```python
from build123d import *

# Parameters (mm, degrees)
F0_R          = 2.5144921482
F0_R_2        = 19.25
F1_DEPTH      = 5
F4_END_RADIUS = 19.25
F4_REACH      = 78.1652482066


with BuildPart() as f1:
    # F0 (on Front) → F1 (new body)
    with BuildSketch(Plane.XZ):
        with BuildLine():
            Line((-27.2, -28.2), (27.2, -28.2))
            ThreePointArc((27.2, -28.2), (27.9071067812, -27.9071067812), (28.2, -27.2))
            Line((28.2, -27.2), (28.2, 27.2))
            ThreePointArc((28.2, 27.2), (27.9071067812, 27.9071067812), (27.2, 28.2))
            Line((27.2, 28.2), (-27.2, 28.2))
            ThreePointArc((-27.2, 28.2), (-27.9071067812, 27.9071067812), (-28.2, 27.2))
            Line((-28.2, 27.2), (-28.2, -27.2))
            ThreePointArc((-28.2, -27.2), (-27.9071067812, -27.9071067812), (-27.2, -28.2))
        make_face()
        with Locations((-23.57, -23.57)):
            Circle(F0_R, mode=Mode.SUBTRACT)
        with Locations((23.57, -23.57)):
            Circle(F0_R, mode=Mode.SUBTRACT)
        with Locations((-23.57, 23.57)):
            Circle(F0_R, mode=Mode.SUBTRACT)
        Circle(F0_R_2, mode=Mode.SUBTRACT)
        with Locations((23.57, 23.57)):
            Circle(F0_R, mode=Mode.SUBTRACT)
    extrude(amount=F1_DEPTH)

    f4_end = (Plane.ZX.offset(-2.5) * Cylinder(F4_END_RADIUS, 316.1669127895, mode=Mode.PRIVATE)).faces().sort_by_distance((-19.25, -2.5, 0))[0]
    # F3 (on face) → F4 (join, up to the whole of a round face its end follows)
    with BuildSketch(Plane(origin=(-28.2, 0, 0), x_dir=(0, -1, 0), z_dir=(-1, 0, 0))):
        Polygon((4.9999998882, -16.2), (4.9999998882, -19.2), (22.1499998882, -19.2), (22.1499998882, -16.2), (21.9999998882, -16.2), (16.7999998882, -16.2), (16.7999998882, -8.8), (22.1499998882, -8.8), (22.1499998882, -5.8), (4.9999998882, -5.8), align=None)
    f4_long = extrude(amount=-F4_REACH, mode=Mode.PRIVATE)
    add(split(f4_long, bisect_by=f4_end, keep=Keep.ALL, mode=Mode.PRIVATE).solids().sort_by_distance((-28.2, -12.347048043, -12.5))[0])

    # F5: F1 across plane


with BuildPart() as f1_1:
    add(f1.part)
    add(f1.part.mirror(Plane.YZ))


solid = f1_1.part
```
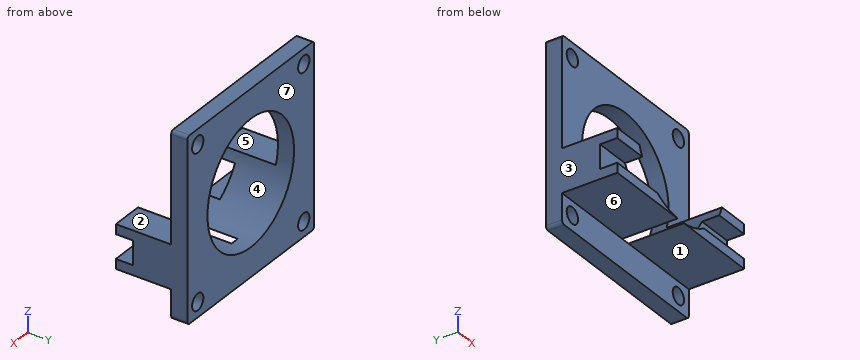
Model file for the job. Use its own axes, mm. Face numbers are marked on the shaded views. A direction names the side the tool comes from. Round coordinates to 2 decimals unless told otherwise and drop trailing zeros. Write each loop counter-clockwise with the first axis right and the second up, starting at its lowest first coordinate (ties: lowest second). Pieces come first, ordered by that corner, then holes. Notation, with made-up numbers: M 61,67 L 68,67 A24 ccw 68,96 Z; hole C 27.5,-17.75 d8. An arc over 180 degrees is marked long. Put each result on its own line as item: value.
Item 1: Cut at B-B (x = 0). List the corners of the cut face in (y, z), and give its area (3 significant figures).
Responses:
outline: M -5,-28.2 L 0,-28.2 L 0,-19.25 L -5,-19.25 Z; M -5,19.25 L 0,19.25 L 0,28.2 L -5,28.2 Z
area: 89.5 mm²
Item 2: Probe L1, parallel to Z at x = -23.57, y = -2.05; L2, parallel to Y at x = 8, z = -20. List the from-to ranges inside material, lowest first. Write a range as from..to.
Responses:
L1: -28.2..-26.08, -21.06..21.06, 26.08..28.2
L2: -5..0
Item 3: Cut at C-C (y = -8.5). List the corners of the cut face in (x, z), and give its area (3 significant figures).
Responses:
outline: M -28.2,-19.2 L -1.39,-19.2 A19.25 cw -18.36,-5.8 L -28.2,-5.8 Z; M 1.39,-19.2 L 28.2,-19.2 L 28.2,-5.8 L 18.36,-5.8 A19.25 cw Z
area: 394 mm²
Item 4: Cut at A-A (z = -23.57). List the corners of the cut face in (x, y).
Responses:
outline: M -28.2,-5 L -26.08,-5 L -26.08,0 L -28.2,0 Z; M -21.06,-5 L 21.06,-5 L 21.06,0 L -21.06,0 Z; M 26.08,-5 L 28.2,-5 L 28.2,0 L 26.08,0 Z
Item 5: Flat gauge pins, fed straight in: P1, Ø1, axis at x = -11, y = -8, coming from the +Z side; P2, Ø1, axis at x = -22, y = -19, coming from the -Z side; P3, Ø4.5, axis at x = 0.5, z = -24.5, coming from the -Y side. Where does each tip first touch, or does it go through?
Responses:
P1: z = -15.44
P2: z = -19.2
P3: y = -5
Item 6: Mould opens along Z. For the marked faces 4, 5, 6 and 7 say: +Z half, -Z half, draft (parallel to the pull), parting line (faces both ways), or undercut.
Responses:
face 4: undercut
face 5: +Z half
face 6: -Z half
face 7: draft
Item 7: Cut at D-D (x = 23.57). List the corners of the cut face in (y, z), and give its area (3 significant figures).
Responses:
outline: M -22.15,-19.2 L -5,-19.2 L -5,-21.06 L 0,-21.06 L 0,21.06 L -5,21.06 L -5,-5.8 L -22.15,-5.8 L -22.15,-8.8 L -16.8,-8.8 L -16.8,-16.2 L -22.15,-16.2 Z; M -5,-28.2 L 0,-28.2 L 0,-26.08 L -5,-26.08 Z; M -5,26.08 L 0,26.08 L 0,28.2 L -5,28.2 Z
area: 422 mm²
Item 8: Tool access for the marked faces 1, 2 and 3: list every direction of +Z, -Z, +X, -X, +Y, -Y with a clear straight run to the whole face (end or side of a thin tool).
Responses:
face 1: -Z, +X, -X, -Y
face 2: +Z, +X, -X, -Y
face 3: +Z, -Z, -X, +Y, -Y
